Design review of the part built by this model. Coordinates are the model's own, in mm. A direction names the side the tool comes from. Coordinates: 2 decimals unless noted, no trailing zeros. Order: outer loops, then holes, each group sorted by start corner. A loop starts at its lowest first (then second) coordinate and runs counter-clockwise, first axis right, second up. Notation, with made-up numbers: M 43.5,89 L 55.5,89 A16 cw 55.5,103 Z; hole C -0.75,61.5 d2. An arc over 180 degrees is marked long. Answer in a Markdown table with one row per item.
from build123d import *

# Parameters (mm, degrees)
SKETCH1_R           = 37.465
BOSS_EXTRUDE1_DEPTH = 3.175
CUT_EXTRUDE1_DEPTH  = 54.078555698
SKETCH3_R           = 2.54
CUT_EXTRUDE2_DEPTH  = 54.078555698
SKETCH4_R           = 1.505
CUT_EXTRUDE3_DEPTH  = 54.078555698


with BuildPart() as part:
    # Sketch1 → Boss-Extrude1 (new body)
    with BuildSketch(Plane.XY):
        Circle(SKETCH1_R)
    extrude(amount=BOSS_EXTRUDE1_DEPTH)

    # Sketch2 → Cut-Extrude1 (cut, through all)
    with BuildSketch(Plane.XY.offset(3.175)):
        with BuildLine():
            Line((-24.593444248, -6.35), (-7.931147458, -6.35))
            ThreePointArc((-7.931147458, -6.35), (0, -10.16), (7.931147458, -6.35))
            Line((7.931147458, -6.35), (24.593444248, -6.35))
            ThreePointArc((24.593444248, -6.35), (0, -25.4), (-24.593444248, -6.35))
        make_face()
        with BuildLine():
            Line((7.931147458, 6.35), (24.593444248, 6.35))
            ThreePointArc((24.593444248, 6.35), (0, 25.4), (-24.593444248, 6.35))
            Line((-24.593444248, 6.35), (-7.931147458, 6.35))
            ThreePointArc((-7.931147458, 6.35), (0, 10.16), (7.931147458, 6.35))
        make_face()
    extrude(amount=-CUT_EXTRUDE1_DEPTH, mode=Mode.SUBTRACT)

    # Sketch3 → Cut-Extrude2 (cut, through all)
    with BuildSketch(Plane.XY.offset(3.175)):
        Circle(SKETCH3_R)
    extrude(amount=-CUT_EXTRUDE2_DEPTH, mode=Mode.SUBTRACT)

    # Sketch4 → Cut-Extrude3 (cut, through all)
    with BuildSketch(Plane(origin=(0, 0, 0), x_dir=(-1, 0, 0), z_dir=(0, 0, -1))):
        with Locations((-4.699, 0)):
            Circle(SKETCH4_R)
        with Locations((4.699, 0)):
            Circle(SKETCH4_R)
    extrude(amount=-CUT_EXTRUDE3_DEPTH, mode=Mode.SUBTRACT)


solid = part.part
(1) For line 1 along Y through (x, z) = (0, 1.5) (3 decimals); line 2 along Y through (x, z) = (-23, 1.95); line 3 along Y through (x, z) = (9.5, 2.45), list the stretches that pass through material, from the lowest coordinate up. Write a range as from..to.
Return value:
| item | result |
|---|---|
| line 1 | y = -37.465..-25.4, -10.16..-2.54, 2.54..10.16, 25.4..37.465 |
| line 2 | y = -29.57..-10.78, -6.35..6.35, 10.78..29.57 |
| line 3 | y = -36.24..-23.56, -6.35..6.35, 23.56..36.24 |
(2) Add section B-B, the plane z = 1.6. Give the boundary of the cut face in (x, y) (3 decimals), and give its area (3 significant figures).
Return value:
| item | result |
|---|---|
| outline | C 0,0 d74.93; hole M -24.593,-6.35 A25.4 ccw 24.593,-6.35 L 7.931,-6.35 A10.16 cw -7.931,-6.35 Z; hole M -24.593,6.35 L -7.931,6.35 A10.16 cw 7.931,6.35 L 24.593,6.35 A25.4 ccw Z; hole C -4.699,0 d3.01; hole C 0,0 d5.08; hole C 4.699,0 d3.01 |
| area | 3,070 mm2 |
(3) Add section C-C, the plane x = 0. Give the boundary of the cut face in (y, z) (3 decimals), and give its area (3 significant figures).
Return value:
| item | result |
|---|---|
| outline | M -37.465,0 L -25.4,0 L -25.4,3.175 L -37.465,3.175 Z; M -10.16,0 L -2.54,0 L -2.54,3.175 L -10.16,3.175 Z; M 2.54,0 L 10.16,0 L 10.16,3.175 L 2.54,3.175 Z; M 25.4,0 L 37.465,0 L 37.465,3.175 L 25.4,3.175 Z |
| area | 125 mm2 |
(4) Insertion check: pin 1 Ø1 at (x, z) = (13, 1) entering from +Y; pin 2 Ø1 at (x, z) = (6, 2.5) entering from -Y; pin 3 Ø1.6 at (x, z) = (-14.5, 2) entering from -Y. Each pin has a flat end and moves straight along its axis. Give the tip position at first contact, or say it passes through.
Return value:
| item | result |
|---|---|
| pin 1 | stops at y = 35.32 |
| pin 2 | stops at y = -37.06 |
| pin 3 | stops at y = -34.87 |
(5) For faces 1 (the flat face through (8, 1, 3.175)), 2 (the cylindrical face through (-0.13, -10.16, 1.61)), list the 3-axis set-ups (+Z, -Z, +X, -X, +Y, -Y) from which the entire face can be reached by the end or side of a thin tool; tool diameter is ignored.
Return value:
| item | result |
|---|---|
| face 1 | +Z, +X, -X, +Y, -Y |
| face 2 | +Z, -Z |
(6) Add section A-A, the plane y = 0. Give the boundary of the cut face in (x, z) (3 decimals), and give its area (3 significant figures).
Return value:
| item | result |
|---|---|
| outline | M -37.465,0 L -6.204,0 L -6.204,3.175 L -37.465,3.175 Z; M -3.194,0 L -2.54,0 L -2.54,3.175 L -3.194,3.175 Z; M 2.54,0 L 3.194,0 L 3.194,3.175 L 2.54,3.175 Z; M 6.204,0 L 37.465,0 L 37.465,3.175 L 6.204,3.175 Z |
| area | 203 mm2 |
(7) Add section D-D, the plane x = 10.5. Give the boundary of the cut face in (y, z) (3 decimals), and give its area (3 significant figures).
Return value:
| item | result |
|---|---|
| outline | M -35.964,0 L -23.128,0 L -23.128,3.175 L -35.964,3.175 Z; M -6.35,0 L 6.35,0 L 6.35,3.175 L -6.35,3.175 Z; M 23.128,0 L 35.964,0 L 35.964,3.175 L 23.128,3.175 Z |
| area | 122 mm2 |
(8) Draft analysis for pull direction X (two halves, no side actions). For faces 3 (the cylindrical face through (-0.13, 10.16, 1.61)), 4 (the cylindrical face through (-29.73, -22.8, 1.57)), 5 (the flat face through (8, 1, 0)), 6 (the cylindrical face through (0.469, -25.396, 1.61)), state which applies: pulls with the +X half, pulls with the -X half, needs draft (parallel to the pull), parting line crosses it, or undercut.
Return value:
| item | result |
|---|---|
| face 3 | undercut |
| face 4 | parting line crosses it |
| face 5 | needs draft |
| face 6 | undercut |
